The listing builds one solid part. Answer for the finished solid, in the listing's coordinates (mm). A direction names the side the tool comes from. Give positions to 0.01 mm unless a question says otherwise; leave off trailing zeros. Write each loop counter-clockwise with the first axis right and the second up, starting at its lowest first coordinate (ties: lowest second). Pieces come first, ordered by that corner, then holes. Notation, with made-up numbers: (21, -37) - (56, -37) arc R16 ccw to (56, -14) - close; hole circle Ø7 at (45.25, 46.25). An arc over 180 degrees is marked (long way). Answer in a Markdown table with one row per item. Add a question column.
Solid Edge part; units mm, degrees
sketch "Sketch1" plane through (0, 0, 0) normal (0, -1, 0) x (1, 0, 0)
  line L0 (19, 37) -> (-19, 37)
  line L1 (-19, 37) -> (-19, -37)
  line L2 (-19, -37) -> (19, -37)
  line L3 (19, -37) -> (19, 37)
extrude "Protrusion1" add sketch "Sketch1" along normal blind 6.6
hole "Hole_1" at (0, -6.6, 0) direction (0, 1, 0) diameter 3.4 end up to next counterbore diameter 6.5 counterbore depth 3.5
1. Section A-A (x = 0) is taken. Give the vertices of the cut face in (y, z), and give its area (3 significant figures).
2. Section B-B (z = 0) is taken. Give the vertices of the cut face in (x, y).
3. Straight lines are drawn through the part: L1, parallel to X at y = -5.35, z = 0; L2, parallel to X at y = -1.1, z = 0; L3, parallel to Z at x = 0, y = -4.95. For each, find the intervals that lie inside material, in ascending order. Write a range as [from, to].
4. Given pin 1 Ø2.5 at (x, z) = (0, 0) entering from +Y, flat-ended and moving along its own axis, determine where the tip first touches the part or whether it passes through.
5. A tool of negligible diameter and unlimited length cuts with its end or side. For faces 1 (the face through (4, 0, 1)), 2 (the face through (1.978, -4.826, 2.579)), from which of +Z, -Z, +X, -X, +Y, -Y can it reach the whole face along a straight path? Write none if from no direction.
Geometry check:
| question | item | result |
|---|---|---|
| 1 | outline | (-6.6, -37) - (0, -37) - (0, -1.7) - (-3.1, -1.7) - (-3.1, -3.25) - (-6.6, -3.25) - close; (-6.6, 3.25) - (-3.1, 3.25) - (-3.1, 1.7) - (0, 1.7) - (0, 37) - (-6.6, 37) - close |
| 1 | area | 455 mm² |
| 2 | outline | (-19, -6.6) - (-3.25, -6.6) - (-3.25, -3.1) - (-1.7, -3.1) - (-1.7, 0) - (-19, 0) - close; (1.7, -3.1) - (3.25, -3.1) - (3.25, -6.6) - (19, -6.6) - (19, 0) - (1.7, 0) - close |
| 3 | L1 | [-19, -3.25], [3.25, 19] |
| 3 | L2 | [-19, -1.7], [1.7, 19] |
| 3 | L3 | [-37, -3.25], [3.25, 37] |
| 4 | pin 1 | through |
| 5 | face 1 | +Z, -Z, +X, -X, +Y |
| 5 | face 2 | -Y |
